```python
from build123d import *

# Parameters (mm, degrees)
SKETCH_1_W          = 74
SKETCH_1_H          = 20
EXTRUDE_1_DEPTH     = 4.1
SKETCH_2_R          = 2.5
CUT_EXTRUDE_1_DEPTH = 4.1


with BuildPart() as part:
    # 草图1 → 凸台-拉伸1 (new body)
    with BuildSketch(Plane(origin=(0, 0, 0), x_dir=(1, 0, 0), z_dir=(0, 1, 0))):
        with Locations((37, 10)):
            Rectangle(SKETCH_1_W, SKETCH_1_H)
    extrude(amount=EXTRUDE_1_DEPTH)

    # 草图2 → 切除-拉伸1 (cut)
    with BuildSketch(Plane(origin=(0, 4.1, 0), x_dir=(1, 0, 0), z_dir=(0, 1, 0))):
        with Locations(Location((66, 10, 0), (0, 0, 270))):
            Circle(SKETCH_2_R)
        with Locations(Location((51, 10, 0), (0, 0, 270))):
            Circle(SKETCH_2_R)
        with BuildLine():
            Line((14, 12.5), (29, 12.5))
            ThreePointArc((29, 12.5), (31.5, 10), (29, 7.5))
            Line((29, 7.5), (14, 7.5))
            ThreePointArc((14, 7.5), (11.5, 10), (14, 12.5))
        make_face()
    extrude(amount=-CUT_EXTRUDE_1_DEPTH, mode=Mode.SUBTRACT)


solid = part.part
```
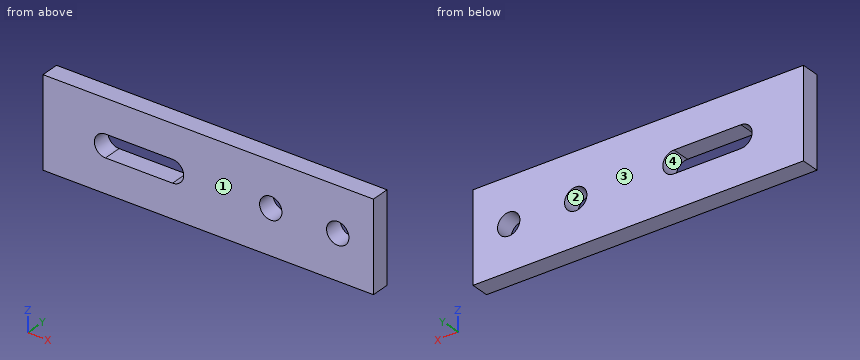
Here's how the part is built. I have some questions about the finished solid (model axes, mm). Face numbers are marked on the shaded views. A direction names the side the tool comes from. Coordinates: 2 decimals unless noted, no trailing zeros. Write each loop counter-clockwise with the first axis right and the second up, starting at its lowest first coordinate (ties: lowest second). Pieces come first, ordered by that corner, then holes. Notation, with made-up numbers: (20.25, -15) - (44.25, -15) arc R19 cw to (44.25, -11) - close; hole circle Ø2 at (-20, 29.5). An arc over 180 degrees is marked (long way). One line per item, written item: value.
1) Suppose I cut it at B-B on y = 1.8. Write out the boundary of the cut face in (x, z), and give its area (3 significant figures).
Model answer:
outline: (0, -20) - (74, -20) - (74, 0) - (0, 0) - close; hole (14, -12.5) - (29, -12.5) arc R2.5 ccw to (29, -7.5) - (14, -7.5) arc R2.5 ccw to start; hole circle Ø5 at (51, -10); hole circle Ø5 at (66, -10)
area: 1,350 mm²
2) Suppose I cut it at C-C on x = 51. Write out the boundary of the cut face in (y, z).
Model answer:
outline: (0, -20) - (4.1, -20) - (4.1, -12.5) - (0, -12.5) - close; (0, -7.5) - (4.1, -7.5) - (4.1, 0) - (0, 0) - close
3) On a 3-axis mill with a long thin cutter (end or side, diameter ignored), from which of +Z, -Z, +X, -X, +Y, -Y can I reach the whole of each face in a straight line? I mean the marked faces 3 and 4. Say none if no direction works.
Model answer:
face 3: +Z, -Z, +X, -X, +Y
face 4: +Y, -Y
4) I need wall thicknesses on line 1 along X through (y, z) = (1.4, -10); line 2 along X through (y, z) = (0.95, -11); line 3 along Z through (x, y) = (64.5, 1). Which ranges of each line are inside material? Lowest first, please.
Model answer:
line 1: x = 0 to 11.5, 31.5 to 48.5, 53.5 to 63.5, 68.5 to 74
line 2: x = 0 to 11.71, 31.29 to 48.71, 53.29 to 63.71, 68.29 to 74
line 3: z = -20 to -12, -8 to 0
5) Suppose I cut it at A-A on z = -10. Write out the boundary of the cut face in (x, y), and give its area (3 significant figures).
Model answer:
outline: (0, 0) - (11.5, 0) - (11.5, 4.1) - (0, 4.1) - close; (31.5, 0) - (48.5, 0) - (48.5, 4.1) - (31.5, 4.1) - close; (53.5, 0) - (63.5, 0) - (63.5, 4.1) - (53.5, 4.1) - close; (68.5, 0) - (74, 0) - (74, 4.1) - (68.5, 4.1) - close
area: 180 mm²
6) We'd pull the mould along Z, two halves only. Please class the marked faces 1 and 2: pulls with the +Z half, pulls with the -Z half, needs draft (parallel to the pull), parting line crosses it, or undercut.
Model answer:
face 1: needs draft
face 2: undercut
